The listing builds one solid part. Answer for the finished solid, in the listing's coordinates (mm). Face numbers are marked on the shaded views. Give positions to 0.01 mm unless a question says otherwise; leave off trailing zeros. Loops run counter-clockwise (first coordinate to the right, second up) from the corner with the lowest first, then second, coordinate; pieces in that order, holes last. Notation, with made-up numbers: M -24.75,49.25 L 22.25,49.25 A22 cw 22.25,58.25 Z; hole C 72,-31 d9. An arc over 180 degrees is marked long. One line per item, written item: value. Start each with the question number.
Q1. A cutting plane is placed at B-B, the plane x = 70. Determine the outline of the cut face in (y, z), and give its area (3 significant figures).
Q2. Consider L1, parallel to Z at x = 111, y = 0 (3 decimals); L2, parallel to Y at x = 114.5, z = -17; L3, parallel to Y at x = 1, z = 0. Determine where each line is inside the solid, lowest interval first.
Q3. A cutting plane is placed at A-A, the plane x = 131.5. Determine the outline of the cut face in (y, z) (3 decimals), and give its area (3 significant figures).
Q4. The mould has two halves that part along Y. Classify the marked faces 1 and 2: +Y half, -Y half, draft (parallel to the pull), parting line (faces both ways), or undercut.
Q5. Flat-ended cylindrical pins translate along their axes: pin 1 (10 mm diameter, centred on x = 91, y = -17.5, fed in from +Z); pin 2 (7.5 mm diameter, centred on y = 0, z = 0, fed in from +X); pin 3 (8 mm diameter, centred on x = 114.5, y = 4.5, fed in from +Z); pin 4 (8 mm diameter, centred on y = -4.5, z = 3.5, fed in from -X). Find the tip coordinate at first contact, or state that the pin passes through.
from build123d import *

# Parameters (mm, degrees)
FILLET1_R                    = 1.5494
F_0_257_DIAMETER_HOLE1_D     = 6.5278
F_0_257_DIAMETER_HOLE1_DEPTH = 13.913851026
F_0_257_DIAMETER_HOLE1_TIP   = 1.961148974
FILLET2_R                    = 0.508
SKETCH4_R                    = 7.366
CUT_EXTRUDE1_DEPTH           = 24.13
CUT_EXTRUDE1_TAPER           = -15
FILLET3_R                    = 0.254
CUT_EXTRUDE2_REACH           = 153.771
SKETCH5_R                    = 8.0264


with BuildPart() as part:
    # Sketch1 → Revolve1 (revolve)
    with BuildSketch(Plane.XY):
        Polygon((25.310022167, 15.9385), (96.398972647, 28.4734), (97.160972647, 28.4734), (97.160972647, 27.305), (151.770972647, 27.305), (151.770972647, 26.035), (91.346485275, 26.035), (27.94, 14.854725894), (27.94, 0), (0, 0), (0, 8.7376), (25.310022167, 15.5194), align=None)
    revolve(axis=Axis((0, 0, 0), (1, 0, 0)))

    # Fillet1
    fillet1_edges = [part.edges().sort_by_distance(p)[0] for p in [
        (27.94, -14.854725894, 0),
    ]]
    fillet(fillet1_edges, radius=FILLET1_R)

    # F (0.257) Diameter Hole1
    with Locations(Plane(origin=(27.94, 0, 0), x_dir=(0, 0, -1), z_dir=(1, 0, 0))):
        with Locations((0, 0)):
            Hole(F_0_257_DIAMETER_HOLE1_D / 2, depth=F_0_257_DIAMETER_HOLE1_DEPTH)
            with Locations((0, 0, -(F_0_257_DIAMETER_HOLE1_DEPTH + F_0_257_DIAMETER_HOLE1_TIP / 2))):  # 118° drill point
                Cone(0, F_0_257_DIAMETER_HOLE1_D / 2, F_0_257_DIAMETER_HOLE1_TIP, mode=Mode.SUBTRACT)

    # Fillet2
    fillet2_edges = [part.edges().sort_by_distance(p)[0] for p in [
        (0, -8.7376, 0),
    ]]
    fillet(fillet2_edges, radius=FILLET2_R)

    # Sketch4 → Cut-Extrude1 (cut)
    with BuildSketch(Plane.ZY):
        Circle(SKETCH4_R)
    extrude(amount=-CUT_EXTRUDE1_DEPTH, taper=CUT_EXTRUDE1_TAPER, mode=Mode.SUBTRACT)

    # Fillet3
    fillet3_edges = [part.edges().sort_by_distance(p)[0] for p in [
        (24.13, 0, -13.831614013),
    ]]
    fillet(fillet3_edges, radius=FILLET3_R)

    # Sketch5 → Cut-Extrude2 (cut, up to next)
    with BuildSketch(Plane(origin=(0, 0, 0), x_dir=(0, 0, -1), z_dir=(1, 0, 0)), mode=Mode.PRIVATE) as cut_extrude2_sk1:
        Circle(SKETCH5_R)
    cut_extrude2_tool1 = extrude(cut_extrude2_sk1.sketch, amount=CUT_EXTRUDE2_REACH, mode=Mode.PRIVATE) & part.part
    add(cut_extrude2_tool1.solids().sort_by_distance((0, 0, 0))[0], mode=Mode.SUBTRACT)


solid = part.part
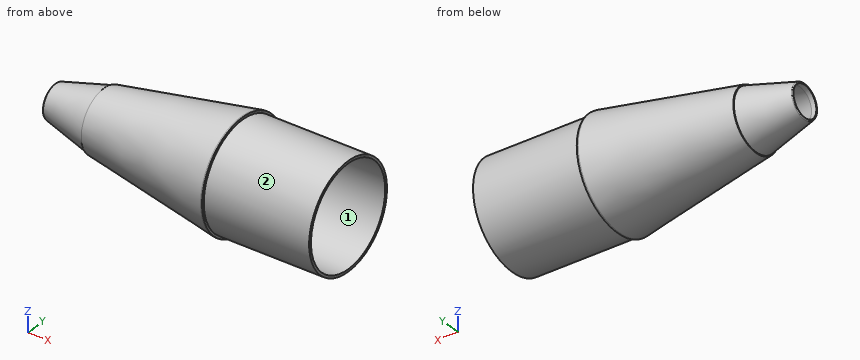
Answer block:
1. outline: C 0,0 d47.64; hole C 0,0 d44.54
1. area: 224 mm^2
2. L1: -27.305 to -26.035, 26.035 to 27.305
2. L2: -21.37 to -19.72, 19.72 to 21.37
2. L3: -9.01 to -8.03, 8.03 to 9.01
3. outline: C 0,0 d54.61; hole C 0,0 d52.07
3. area: 213 mm^2
4. face 1: undercut
4. face 2: parting line
5. pin 1: z = 24.7
5. pin 2: x = 27.94
5. pin 3: z = 27.3
5. pin 4: x = 0
